Read the model definition and answer for the solid it produces. Units are mm, in the model's axes. A direction names the side the tool comes from. Coordinates: 2 decimals unless noted, no trailing zeros. Loops run counter-clockwise (first coordinate to the right, second up) from the corner with the lowest first, then second, coordinate; pieces in that order, holes last. Notation, with made-up numbers: (46, -33.75) - (94, -33.75) arc R15 cw to (94, -15.75) - close; hole circle Ø3 at (-12.5, 32). An arc over 180 degrees is marked (long way). Use CSV: the item, a comma, the result in double quotes.
```python
from build123d import *

# Parameters (mm, degrees)
SKETCH_W        = 96
SKETCH_H        = 116
PAD_DEPTH       = 2
SKETCH001_R     = 1.3
POCKET_DEPTH    = 2.001
CHAMFER_SIZE    = 1.1
SKETCH003_W     = 25
SKETCH003_H     = 50
PAD001_DEPTH    = 11
SKETCH004_W     = 25
SKETCH004_H     = 13
PAD002_DEPTH    = 2
POCKET001_DEPTH = 8.8
SKETCH008_W     = 12.5
SKETCH008_H     = 12
POCKET004_DEPTH = 1.3
SKETCH009_W     = 37.451334
SKETCH009_H     = 40.177643
POCKET005_DEPTH = 7
SKETCH010_W     = 12
SKETCH010_H     = 1.2
PAD003_DEPTH    = 12.5
SKETCH011_W     = 2
SKETCH011_H     = 3.8
PAD004_DEPTH    = 8
POCKET006_DEPTH = 60.155704
PAD005_DEPTH    = 8
SKETCH015_W     = 5.7
SKETCH015_H     = 11.2
PAD006_DEPTH    = 1.2
SKETCH016_W     = 31
SKETCH016_H     = 31
PAD007_DEPTH    = 2
SKETCH017_W     = 82
SKETCH017_H     = 2
PAD008_DEPTH    = 3
PAD009_DEPTH    = 28
PAD010_DEPTH    = 28
SKETCH020_W     = 2
SKETCH020_H     = 99
PAD011_DEPTH    = 4


with BuildPart() as part:
    # Sketch → Pad (new body)
    with BuildSketch(Plane.XY):
        with Locations((0, 58)):
            Rectangle(SKETCH_W, SKETCH_H)
    extrude(amount=PAD_DEPTH)

    # Sketch001 (on Face6 of Pad) → Pocket (cut, through all)
    with BuildSketch(Plane.XY.offset(2)):
        with Locations((-45.5, 113.5)):
            Circle(SKETCH001_R)
        with Locations((45.5, 113.5)):
            Circle(SKETCH001_R)
        with Locations((45.5, 2.5)):
            Circle(SKETCH001_R)
        with Locations((-45.5, 2.5)):
            Circle(SKETCH001_R)
    extrude(amount=-POCKET_DEPTH, mode=Mode.SUBTRACT)

    # Chamfer
    chamfer_edges = [part.edges().sort_by_distance(p)[0] for p in [
        (-46.8, 113.5, 2),
        (44.2, 113.5, 2),
        (44.2, 2.5, 2),
        (-46.8, 2.5, 2),
    ]]
    chamfer(chamfer_edges, length=CHAMFER_SIZE)

    # Sketch003 → Pad001 (join)
    with BuildSketch(Plane(origin=(0, 0, 0), x_dir=(1, 0, 0), z_dir=(0, 0, -1))):
        with Locations((-0.345296, -91)):
            Rectangle(SKETCH003_W, SKETCH003_H)
    extrude(amount=PAD001_DEPTH)

    # Sketch004 (on Face12 of Pad001) → Pad002 (join)
    with BuildSketch(Plane(origin=(0, 116, 0), x_dir=(-1, 0, 0), z_dir=(0, 1, 0))):
        with Locations((0.345296, -4.5)):
            Rectangle(SKETCH004_W, SKETCH004_H)
    extrude(amount=PAD002_DEPTH)

    # Sketch005 (on Face24 of Pad002) → Pocket001 (cut)
    with BuildSketch(Plane(origin=(0, 0, -11), x_dir=(1, 0, 0), z_dir=(0, 0, -1))):
        Polygon((-9.75, -69), (-9.75, -104), (-4, -104), (-4, -106), (-6.25, -106), (-6.25, -118), (6.25, -118), (6.25, -106), (4, -106), (4, -104), (9.75, -104), (9.75, -69), (5.5, -69), (5.5, -70.3), (3.5, -70.3), (3.5, -69), (-3.5, -69), (-3.5, -70.3), (-5.5, -70.3), (-5.5, -69), align=None)
    extrude(amount=-POCKET001_DEPTH, mode=Mode.SUBTRACT)

    # Sketch008 (on Face26 of Pocket001) → Pocket004 (cut)
    with BuildSketch(Plane(origin=(0, 0, -2.2), x_dir=(1, 0, 0), z_dir=(0, 0, -1))):
        with Locations((0, -112)):
            Rectangle(SKETCH008_W, SKETCH008_H)
    extrude(amount=-POCKET004_DEPTH, mode=Mode.SUBTRACT)

    # Sketch009 (on Face24 of Pocket004) → Pocket005 (cut)
    with BuildSketch(Plane(origin=(0, 0, -11), x_dir=(1, 0, 0), z_dir=(0, 0, -1))):
        with Locations((-0.643557, -83.911179)):
            Rectangle(SKETCH009_W, SKETCH009_H)
    extrude(amount=-POCKET005_DEPTH, mode=Mode.SUBTRACT)

    # Sketch010 (on Face29 of Pocket005) → Pad003 (join)
    with BuildSketch(Plane.YZ.offset(-6.25)):
        with Locations((112, -10.4)):
            Rectangle(SKETCH010_W, SKETCH010_H)
    extrude(amount=PAD003_DEPTH)

    # Sketch011 (on Face51 of Pad003) → Pad004 (join)
    with BuildSketch(Plane.YZ.offset(-4)):
        with Locations((105, -9.1)):
            Rectangle(SKETCH011_W, SKETCH011_H)
    extrude(amount=PAD004_DEPTH)

    # Sketch012 (on Face23 of Pad004) → Pocket006 (cut, through all)
    with BuildSketch(Plane.YZ.offset(12.154704)):
        Polygon((118, 2), (113.889458, -14.486482), (118, -14.486482), align=None)
    extrude(amount=-POCKET006_DEPTH, mode=Mode.SUBTRACT)

    # Sketch014 (on Face4 of Pocket006) → Pad005 (join)
    with BuildSketch(Plane(origin=(0, 0, 0), x_dir=(1, 0, 0), z_dir=(0, 0, -1))):
        Polygon((-4.85, -42.8), (4.85, -42.8), (4.85, -54), (6.85, -54), (6.85, -63), (4.85, -63), (4.85, -56), (2.85, -56), (2.85, -44.8), (-2.85, -44.8), (-2.85, -49.2), (-3.45, -49.2), (-3.45, -51), (-2.85, -51), (-2.85, -56), (-4.85, -56), (-4.85, -63), (-6.85, -63), (-6.85, -54), (-4.85, -54), align=None)
    extrude(amount=PAD005_DEPTH)

    # Sketch015 (on Face4 of Pad005) → Pad006 (join)
    with BuildSketch(Plane(origin=(0, 0, 0), x_dir=(1, 0, 0), z_dir=(0, 0, -1))):
        with Locations((0, -50.4)):
            Rectangle(SKETCH015_W, SKETCH015_H)
    extrude(amount=PAD006_DEPTH)

    # Sketch016 (on Face4 of Pad006) → Pad007 (join)
    with BuildSketch(Plane(origin=(0, 0, 0), x_dir=(1, 0, 0), z_dir=(0, 0, -1))):
        with Locations((27.654704, -81.5)):
            Rectangle(SKETCH016_W, SKETCH016_H)
        Polygon((14.154704, -68), (14.154704, -81), (15.154704, -81), (15.154704, -82), (14.154704, -82), (14.154704, -95), (27.154704, -95), (27.154704, -94), (28.154704, -94), (28.154704, -95), (41.154704, -95), (41.154704, -82), (40.154704, -82), (40.154704, -81), (41.154704, -81), (41.154704, -68), (28.154704, -68), (28.154704, -69), (27.154704, -69), (27.154704, -68), align=None, mode=Mode.SUBTRACT)
    extrude(amount=PAD007_DEPTH)

    # Sketch017 (on Face4 of Pad007) → Pad008 (join)
    with BuildSketch(Plane(origin=(0, 0, 0), x_dir=(1, 0, 0), z_dir=(0, 0, -1))):
        with Locations((0, -1)):
            Rectangle(SKETCH017_W, SKETCH017_H)
    extrude(amount=PAD008_DEPTH)

    # Sketch018 (on Face10 of Pad008) → Pad009 (join)
    with BuildSketch(Plane.YZ.offset(12.154704)):
        Polygon((116, 0), (112.758736, -11), (110.758736, -11), (114, 0), align=None)
    extrude(amount=PAD009_DEPTH)

    # Sketch019 (on Face17 of Pad009) → Pad010 (join)
    with BuildSketch(Plane(origin=(-12.845296, 0, 0), x_dir=(0, -1, 0), z_dir=(-1, 0, 0))):
        Polygon((-116, 0), (-112.758736, -11), (-110.758736, -11), (-114, 0), align=None)
    extrude(amount=PAD010_DEPTH)

    # Sketch020 (on Face4 of Pad010) → Pad011 (join)
    with BuildSketch(Plane(origin=(0, 0, 0), x_dir=(1, 0, 0), z_dir=(0, 0, -1))):
        with Locations((-47, -56.5)):
            Rectangle(SKETCH020_W, SKETCH020_H)
        with Locations((47, -56.5)):
            Rectangle(SKETCH020_W, SKETCH020_H)
    extrude(amount=PAD011_DEPTH)


solid = part.part
```
Q1. For a pull along Z with two mould halves and no side action, classify faces 1 (the face through (25.959, 112.357, -5.577)), 2 (the face through (44.542, 114.379, 0.456)), 3 (the face through (14, 81, -2)), 4 (the face through (0, 112, -0.9)) as +Z half, -Z half, draft (parallel to the pull), parting line (faces both ways), or undercut.
Reported:
face 1,"undercut"
face 2,"draft"
face 3,"-Z half"
face 4,"undercut"
Q2. Find the intervals of material crossed by probe 1 along Y at (x, z) = (45.5, 0.3); probe 2 along X at (y, z) = (113.5, 0.4); probe 3 along X at (y, z) = (73.5, -2.75), in increasing order. Write a range as [from, to].
Reported:
probe 1,"y = [0, 1.2], [3.8, 112.2], [114.8, 116]"
probe 2,"x = [-48, -46.8], [-44.2, 44.2], [46.8, 48]"
probe 3,"x = [-48, -46], [-12.85, -9.75], [9.75, 12.15], [46, 48]"
Q3. Given P1, Ø1, axis at x = -26, z = 1.5, coming from the +Y side; P2, Ø7.5, axis at x = -1.5, y = 90.5, coming from the -Z side; P3, Ø15, axis at x = -0.5, y = 56, coming from the -Z side; P4, Ø1.6, axis at x = -45.5, y = 2.5, coming from the -Z side, each flat-ended and moving along its own axis, determine where each tip first touches the part or whether it passes through.
Reported:
P1,"stops at y = 116"
P2,"stops at z = -2.2"
P3,"stops at z = -8"
P4,"passes through"
Q4. A tool of negligible diameter and unlimited length cuts with its end or side. For faces 5 (the face through (12.155, 116, -5)), 6 (the face through (-2.85, 53, -5)), 7 (the face through (-46, 57, -2)), from which of +Z, -Z, +X, -X, +Y, -Y can it reach the whole face along a straight path? Write none if from no direction.
Reported:
face 5,"-Z, +X, +Y"
face 6,"-Z"
face 7,"-Z, +Y, -Y"
Q5. The part is cut by section A-A on y = 37.5. Determine the outline of the cut face in (x, z), and give its area (3 significant figures).
Reported:
outline,"(-48, -4) - (-46, -4) - (-46, 0) - (46, 0) - (46, -4) - (48, -4) - (48, 2) - (-48, 2) - close"
area,"208 mm²"
